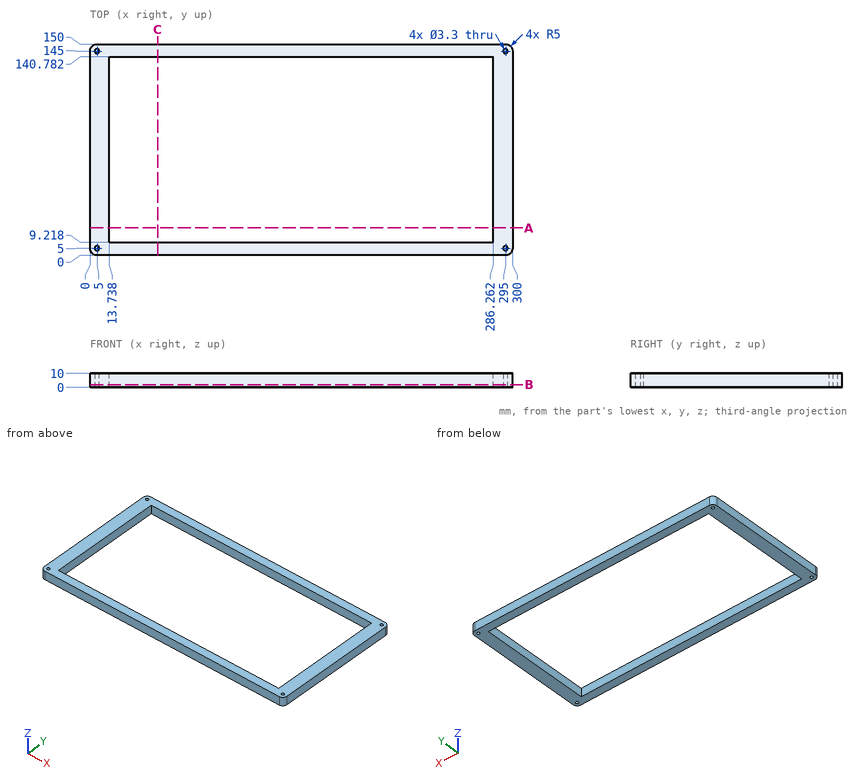
Drawing for the job (mm, zero at the part's lowest x, y, z). Round coordinates to 2 decimals unless told otherwise and drop trailing zeros. Order: outer loops, then holes, each group sorted by start corner. A loop starts at its lowest first (then second) coordinate and runs counter-clockwise, first axis right, second up.
Item 1: Probe line 1 along X through (y, z) = (145, 4.25); line 2 along Y through (x, z) = (5, 5.75); line 3 along Y through (x, z) = (46.5, 2.5). List the from-to ranges inside material, lowest first.
Item 2: Saw through at A-A on y = 19.5. Write the cut outline in (x, z).
Item 3: Pin check, flat tip, straight feed: pin 1 (3 mm diameter, centred on x = 295, y = 5, fed in from -Z). Stop position of the tip, or through.
Item 4: Saw through at B-B on z = 2. Write the cut outline in (x, y).
Item 5: Saw through at C-C on x = 48. Write the cut outline in (y, z).
Reported:
1. line 1: x = 0 to 3.35, 6.65 to 293.35, 296.65 to 300
1. line 2: y = 0 to 3.35, 6.65 to 143.35, 146.65 to 150
1. line 3: y = 0 to 9.22, 140.78 to 150
2. outline: (0, 0) - (13.74, 0) - (13.74, 10) - (0, 10) - close; (286.26, 0) - (300, 0) - (300, 10) - (286.26, 10) - close
3. pin 1: passes through
4. outline: (0, 5) arc R5 ccw to (5, 0) - (295, 0) arc R5 ccw to (300, 5) - (300, 145) arc R5 ccw to (295, 150) - (5, 150) arc R5 ccw to (0, 145) - close; hole circle Ø3.3 at (5, 5); hole circle Ø3.3 at (5, 145); hole (13.74, 9.22) - (286.26, 9.22) - (286.26, 140.78) - (13.74, 140.78) - close; hole circle Ø3.3 at (295, 5); hole circle Ø3.3 at (295, 145)
5. outline: (0, 0) - (9.22, 0) - (9.22, 10) - (0, 10) - close; (140.78, 0) - (150, 0) - (150, 10) - (140.78, 10) - close
